```python
from build123d import *

# Parameters (mm, degrees)
EXTRUDE_1_DEPTH              = 42
CUT_EXTRUDE_1_DEPTH          = 38
HOLE_WIZARD_M5_1_D           = 4.2
HOLE_WIZARD_M5_1_CSINK_D     = 5.05
HOLE_WIZARD_M5_1_CSINK_ANGLE = 90
PATTERN_CIRCULAR_1_COUNT     = 4


with BuildPart() as part:
    # 草图1 → 凸台-拉伸1 (new body)
    with BuildSketch(Plane.XY):
        with BuildLine():
            Line((-42, 62.136945532), (-42, 80))
            Line((-42, 80), (42, 80))
            Line((42, 80), (42, 62.136945532))
            ThreePointArc((42, 62.136945532), (0, -75), (-42, 62.136945532))
        make_face()
    extrude(amount=EXTRUDE_1_DEPTH)

    # 草图2 → 切除-拉伸1 (cut)
    with BuildSketch(Plane.XY.offset(42)):
        with BuildLine():
            Line((-30, 66.932802123), (-30, 68))
            Line((-30, 68), (30, 68))
            Line((30, 68), (30, 66.932802123))
            ThreePointArc((30, 66.932802123), (30.849629548, 63.854867066), (33.157894737, 61.648633534))
            ThreePointArc((33.157894737, 61.648633534), (58.493479839, 38.451434516), (69.742857143, 5.994487263))
            ThreePointArc((69.742857143, 5.994487263), (64, 0), (69.742857143, -5.994487263))
            ThreePointArc((69.742857143, -5.994487263), (49.497474683, -49.497474683), (5.994487263, -69.742857143))
            ThreePointArc((5.994487263, -69.742857143), (0, -64), (-5.994487263, -69.742857143))
            ThreePointArc((-5.994487263, -69.742857143), (-49.497474683, -49.497474683), (-69.742857143, -5.994487263))
            ThreePointArc((-69.742857143, -5.994487263), (-64, 0), (-69.742857143, 5.994487263))
            ThreePointArc((-69.742857143, 5.994487263), (-58.493479839, 38.451434516), (-33.157894737, 61.648633534))
            ThreePointArc((-33.157894737, 61.648633534), (-30.849629548, 63.854867066), (-30, 66.932802123))
        make_face()
    extrude(amount=-CUT_EXTRUDE_1_DEPTH, mode=Mode.SUBTRACT)

    # M5 螺纹孔1 (through all)
    with Locations(Plane.XY.offset(42)):
        with Locations((0, -68)):
            hole_wizard_m5_1 = CounterSinkHole(HOLE_WIZARD_M5_1_D / 2, HOLE_WIZARD_M5_1_CSINK_D / 2, counter_sink_angle=HOLE_WIZARD_M5_1_CSINK_ANGLE)

    # 阵列(圆周)1: M5 螺纹孔1 ×4 about axis, 1 skipped
    pattern_circular_1_axis = Axis((0, 0, 0), (0, 0, -1))
    add([hole_wizard_m5_1.rotate(pattern_circular_1_axis, i * 360 / PATTERN_CIRCULAR_1_COUNT) for i in range(1, PATTERN_CIRCULAR_1_COUNT) if i not in (2,)], mode=Mode.SUBTRACT)


solid = part.part
```
Can you work these out from the model? Positions are in its coordinate system, mm. A direction names the side the tool comes from. Coordinates: 2 decimals unless noted, no trailing zeros. Loops run counter-clockwise (first coordinate to the right, second up) from the corner with the lowest first, then second, coordinate; pieces in that order, holes last. Notation, with made-up numbers: (-34, 16.25) - (9, 16.25) arc R27 cw to (9, 53.25) - close; hole circle Ø7 at (19.25, 4). An arc over 180 degrees is marked (long way). Answer as CSV lines item,"result". Start each with the question number.
1) I need wall thicknesses on line 1 (Z direction, x = -29.5, y = 39); line 2 (Y direction, x = 54.5, z = 30); line 3 (Y direction, x = -50.5, z = 10). Which ranges of each line are inside material? Lowest first, please. Write a range as from..to.
2) Suppose I cut it at A-A (z = 25.5). Please give me the cut outline in (x, y), plus the area to 3 significant figures.
3) Thinking about a two-plate mould opening in X: for faces 4 (the cylindrical face through (58.225, 38.857, 23.266)), 5 (the flat face through (1, 4, 0)), 6 (the flat face through (-42, 71, 21)), which applies, pulls with the +X half, pulls with the -X half, needs draft (parallel to the pull), parting line crosses it, or undercut?
4) Suppose I cut it at B-B (x = 0). Please give me the cut outline in (y, z) (3 decimals).
5) For pin 1 (8 mm diameter, centred on x = -4.5, z = 18.5, fed in from -Y); pin 2 (0.9 mm diameter, centred on y = 67.5, z = 16, fed in from +X); pin 3 (8 mm diameter, centred on y = 26.5, z = 32, fed in from +X); pin 4 (3.5 mm diameter, centred on x = 0, y = -68, fed in from +Z), each with a flat end and sliding along its axis, tell me the tip position at first contact or that it passes through.
6) Suppose I cut it at C-C (x = -16). Please give me the cut outline in (y, z).
7) Suppose I cut it at D-D (y = 30). Please give me the cut outline in (x, z), plus the area to 3 significant figures.
8) Which directions (+Z, -Z, +X, -X, +Y, -Y) give clear straight access to the entire face, cutting with the end or side of a thin tool? Please do faces 1 (the cylindrical face through (-58.76, 38.04, 23.27)), 2 (the flat face through (-1, 80, 21)), 3 (the flat face through (42, 71, 21)).
Check result:
1,line 1,"z = 0..4"
1,line 2,"y = -51.52..-43.93, 43.93..51.52"
1,line 3,"y = -55.45..-48.47, 48.47..55.45"
2,outline,"(-42, 62.14) arc R75 ccw (long way) to (42, 62.14) - (42, 80) - (-42, 80) - close; hole circle Ø4.2 at (-68, 0); hole (-69.74, -5.99) arc R70 ccw to (-5.99, -69.74) arc R6 cw to (5.99, -69.74) arc R70 ccw to (69.74, -5.99) arc R6 cw to (69.74, 5.99) arc R70 ccw to (33.16, 61.65) arc R6 cw to (30, 66.93) - (30, 68) - (-30, 68) - (-30, 66.93) arc R6 cw to (-33.16, 61.65) arc R70 ccw to (-69.74, 5.99) arc R6 cw to start; hole circle Ø4.2 at (0, -68); hole circle Ø4.2 at (68, 0)"
2,area,"3,150 mm²"
3,face 4,"undercut"
3,face 5,"needs draft"
3,face 6,"pulls with the -X half"
4,outline,"(-75, 0) - (-70.1, 0) - (-70.1, 41.575) - (-70.525, 42) - (-75, 42) - close; (-65.9, 0) - (80, 0) - (80, 42) - (68, 42) - (68, 4) - (-64, 4) - (-64, 42) - (-65.475, 42) - (-65.9, 41.575) - close"
5,pin 1,"stops at y = -75"
5,pin 2,"stops at x = 42"
5,pin 3,"stops at x = 71.55"
5,pin 4,"passes through"
6,outline,"(-73.27, 0) - (80, 0) - (80, 42) - (68, 42) - (68, 4) - (-68.15, 4) - (-68.15, 42) - (-73.27, 42) - close"
7,outline,"(-68.74, 0) - (68.74, 0) - (68.74, 42) - (63.25, 42) - (63.25, 4) - (-63.25, 4) - (-63.25, 42) - (-68.74, 42) - close"
7,area,"967 mm²"
8,face 1,"+Z"
8,face 2,"+Z, -Z, +X, -X, +Y"
8,face 3,"+Z, -Z, +X, +Y"
